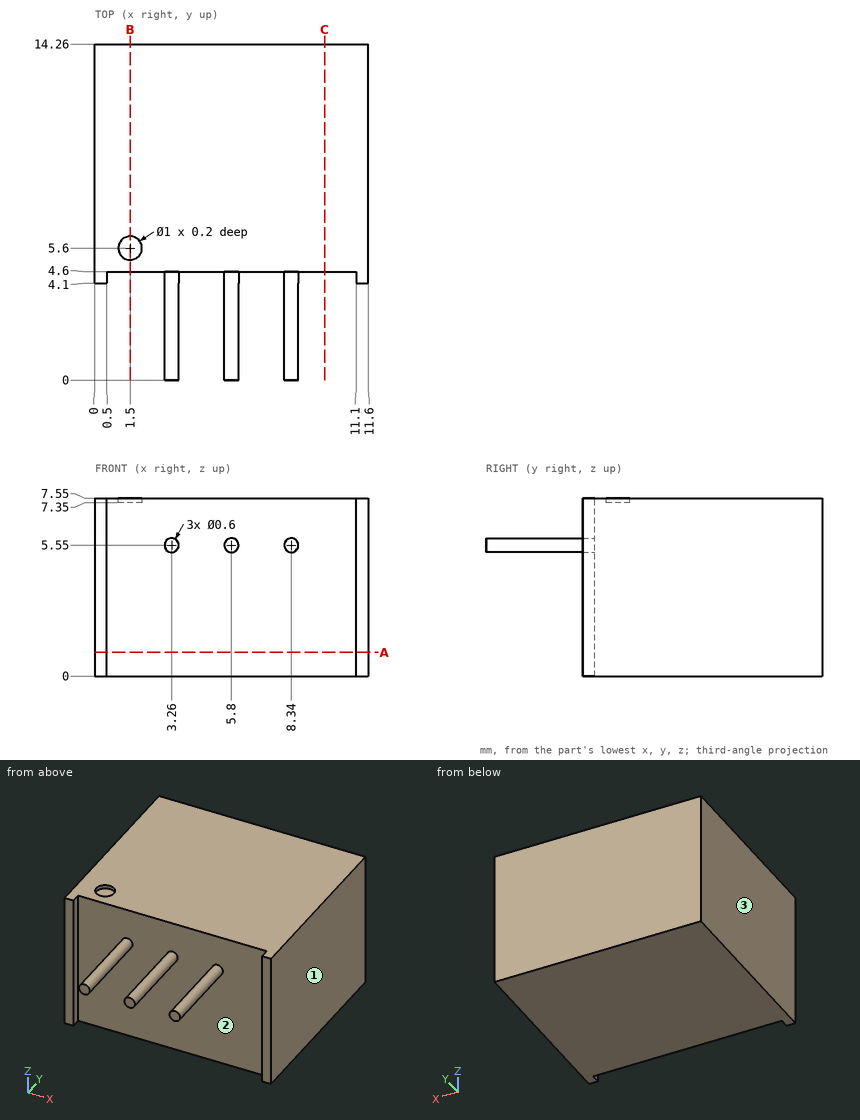
Geometry: see drawing. Coordinates: mm, zero at the bounding-box minimum. Give positions to 0.01 mm unless a question says otherwise; leave off trailing zeros. Order: outer loops, then holes, each group sorted by start corner. A loop starts at its lowest first (then second) coordinate and runs counter-clockwise, first axis right, second up. Notation, with made-up numbers: M 71.25,11 L 96.25,11 A30 cw 96.25,42 Z; hole C 43.5,49 d8. An arc over 180 degrees is marked long. Answer as CSV lines item,"result". Start each with the question number.
1) Cut plane A-A (z = 1). Output: boundary loops of the cut face in (x, y).
2) Mould query, pull axis X, two halves, no side actions, for the marked faces 1, 2 and 3. Classes: +X half, -X half, draft (parallel to the pull), parting line (faces both ways), or undercut.
3) Cut plane B-B (x = 1.5). Output: boundary loops of the cut face in (y, z).
4) First-contact query: P1, Ø2, axis at x = 4, y = 2, coming from the +Z side. Flat tip, straight axial feed; report the tip coordinate or a pass-through.
5) Line query: line 1 (Y direction, x = 1.5, z = 7.5); line 2 (Y direction, x = 9, z = 4.75); line 3 (Y direction, x = 11.25, z = 0.75). Output: solid intervals per line, ascending. Write a range as from..to.
6) Cut plane C-C (x = 9.75). Output: boundary loops of the cut face in (y, z), then the cut area to 3 significant figures.
Findings below:
1,outline,"M 0,4.1 L 0.5,4.1 L 0.5,4.6 L 11.1,4.6 L 11.1,4.1 L 11.6,4.1 L 11.6,14.26 L 0,14.26 Z"
2,face 1,"+X half"
2,face 2,"undercut"
2,face 3,"-X half"
3,outline,"M 4.6,0 L 14.26,0 L 14.26,7.55 L 6.1,7.55 L 6.1,7.35 L 5.1,7.35 L 5.1,7.55 L 4.6,7.55 Z"
4,P1,"stops at z = 5.85"
5,line 1,"y = 4.6..5.1, 6.1..14.26"
5,line 2,"y = 4.6..14.26"
5,line 3,"y = 4.1..14.26"
6,outline,"M 4.6,0 L 14.26,0 L 14.26,7.55 L 4.6,7.55 Z"
6,area,"72.9 mm²"
